from build123d import *

# Parameters (mm, degrees)
F1_DEPTH = 45.2
F2_W     = 26.5
F2_H     = 2
F3_DEPTH = 18.001
F4_DEPTH = 13.848382
F6_DEPTH = 3.2


with BuildPart() as f1:
    # F0 (on Top) → F1 (new body)
    with BuildSketch(Plane.XY):
        with BuildLine():
            Line((11.5, 0), (11.5, -13.847382))
            ThreePointArc((11.5, -13.847382), (0, 18), (-11.5, -13.847382))
            Line((-11.5, -13.847382), (-11.5, 0))
            ThreePointArc((-11.5, 0), (0, 11.5), (11.5, 0))
        make_face()
    extrude(amount=F1_DEPTH)

    # F2 (on Front) → F3 (cut, through all)
    with BuildSketch(Plane.XZ):
        Polygon((-13.25, 43.2), (-14.25, 43.2), (-14.25, 37.2), (14.25, 37.2), (14.25, 43.2), (13.25, 43.2), align=None)
        with Locations((0, 44.2)):
            Rectangle(F2_W, F2_H)
    extrude(amount=-F3_DEPTH, mode=Mode.SUBTRACT)

    # F2 (on Front) → F4 (cut, through all)
    with BuildSketch(Plane.XZ):
        Polygon((-13.25, 43.2), (-14.25, 43.2), (-14.25, 37.2), (14.25, 37.2), (14.25, 43.2), (13.25, 43.2), align=None)
        with Locations((0, 44.2)):
            Rectangle(F2_W, F2_H)
    extrude(amount=F4_DEPTH, mode=Mode.SUBTRACT)

    # F5 (on face) → F6 (cut)
    with BuildSketch(Plane(origin=(0, 0, 0), x_dir=(1, 0, 0), z_dir=(0, 0, -1))):
        with BuildLine():
            ThreePointArc((-11.5, 13.847382), (-15.961029, 8.32139), (-17.937391, 1.5))
            Line((-17.937391, 1.5), (-11.5, 1.5))
            Line((-11.5, 1.5), (-11.5, 13.847382))
        make_face()
        with BuildLine():
            ThreePointArc((-17.937391, -1.5), (-12.727922, -12.727922), (-1.5, -17.937391))
            Line((-1.5, -17.937391), (-1.5, -11.401754))
            ThreePointArc((-1.5, -11.401754), (-8.131728, -8.131728), (-11.401754, -1.5))
            Line((-11.401754, -1.5), (-17.937391, -1.5))
        make_face()
        with BuildLine():
            Line((1.5, -11.401754), (1.5, -17.937391))
            ThreePointArc((1.5, -17.937391), (12.727922, -12.727922), (17.937391, -1.5))
            Line((17.937391, -1.5), (11.401754, -1.5))
            ThreePointArc((11.401754, -1.5), (8.131728, -8.131728), (1.5, -11.401754))
        make_face()
        with BuildLine():
            Line((11.5, 1.5), (17.937391, 1.5))
            ThreePointArc((17.937391, 1.5), (15.961029, 8.32139), (11.5, 13.847382))
            Line((11.5, 13.847382), (11.5, 1.5))
        make_face()
    extrude(amount=-F6_DEPTH, mode=Mode.SUBTRACT)


solid = f1.part
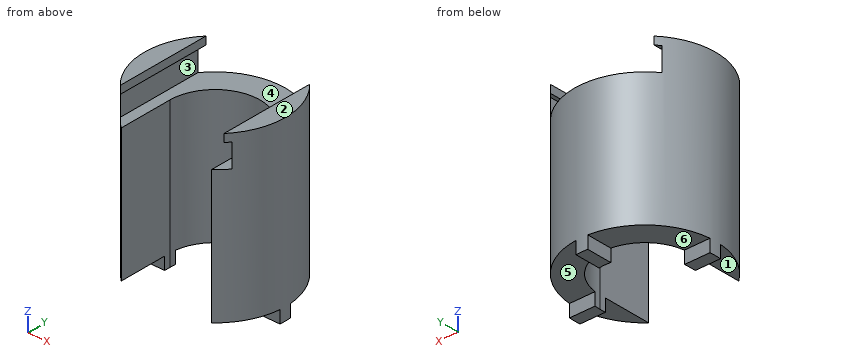
Could you check a few things on this model? Use its own coordinates, in mm. Face numbers are marked on the shaded views. A direction names the side the tool comes from. Coordinates: 2 decimals unless noted, no trailing zeros. Order: outer loops, then holes, each group sorted by start corner. A loop starts at its lowest first (then second) coordinate and runs counter-clockwise, first axis right, second up.
Q1. Suppose I cut it at D-D on x = 16.5. Please give me the cut outline in (y, z).
Q2. Thinking about a two-plate mould opening in Z: for the marked faces 1, 2 and 3, which applies, released by +Z, released by -Z, zero draft, split by the parting line, or undercut?
Q3. Suppose I cut it at A-A on y = 5. Please give me the cut outline in (x, z), and give its area (3 significant figures).
Q4. Suppose I cut it at C-C on z = 25. Please give me the cut outline in (x, y), and give its area (3 significant figures).
Q5. Please list where these lines run through material, in increasing order: L1, parallel to Z at x = 13.5, y = 11; L2, parallel to X at y = -7, z = 30.5; L3, parallel to Z at x = -3.5, y = 12.5.
Q6. Suppose I cut it at B-B on y = 14.5. Please give me the cut outline in (x, z).
Q7. Which directions (+Z, -Z, +X, -X, +Y, -Y) give clear straight access to the entire face, cutting with the end or side of a thin tool? Please do the marked faces 4, 5 and 6.
Q8. Will these pins go through, and if not, where does the flat tip stop? pin 1 (1 mm diameter, centred on y = -0.5, z = 44, fed in from -X); pin 2 (3.5 mm diameter, centred on x = -13.5, z = 1, fed in from -Y); pin 3 (1.9 mm diameter, centred on x = -13.5, y = -7, fed in from -Z); pin 4 (1.6 mm diameter, centred on x = 15, z = 1, fed in from +Y).
Answer:
1. outline: (-7.19, 3.2) - (-1.5, 3.2) - (-1.5, 0) - (1.5, 0) - (1.5, 3.2) - (7.19, 3.2) - (7.19, 45.2) - (-7.19, 45.2) - close
2. face 1: released by -Z
2. face 2: released by +Z
2. face 3: undercut
3. outline: (-17.29, 3.2) - (-10.36, 3.2) - (-10.36, 37.2) - (-14.25, 37.2) - (-14.25, 43.2) - (-13.25, 43.2) - (-13.25, 45.2) - (-17.29, 45.2) - close; (10.36, 3.2) - (17.29, 3.2) - (17.29, 45.2) - (13.25, 45.2) - (13.25, 43.2) - (14.25, 43.2) - (14.25, 37.2) - (10.36, 37.2) - close
3. area: 524 mm2
4. outline: (-11.5, -13.85) - (-11.5, 0) arc R11.5 cw to (11.5, 0) - (11.5, -13.85) arc R18 ccw (long way) to start
4. area: 426 mm2
5. L1: z = 3.2 to 37.2, 43.2 to 45.2
5. L2: x = -16.58 to -11.5, 11.5 to 16.58
5. L3: z = 3.2 to 37.2
6. outline: (-10.67, 3.2) - (-1.5, 3.2) - (-1.5, 0) - (1.5, 0) - (1.5, 3.2) - (10.67, 3.2) - (10.67, 37.2) - (-10.67, 37.2) - close
7. face 4: +Y, -Y
7. face 5: -Z, +X, +Y
7. face 6: -Z, -X, +Y
8. pin 1: stops at x = -18
8. pin 2: stops at y = -1.5
8. pin 3: stops at z = 3.2
8. pin 4: stops at y = 1.5
